from build123d import *

# Parameters (mm, degrees)
ESQUISSE1_R      = 4
EXTRUSION1_DEPTH = 6
CONG_1_R         = 0.5


with BuildPart() as part:
    # Esquisse1 → Extrusion1 (new body)
    with BuildSketch(Plane.XY):
        Polygon((7.505553499, 0), (3.75277675, 6.5), (-3.75277675, 6.5), (-7.505553499, 0), (-3.75277675, -6.5), (3.75277675, -6.5), align=None)
        Circle(ESQUISSE1_R, mode=Mode.SUBTRACT)
    extrude(amount=EXTRUSION1_DEPTH)

    # Congé1
    cong_1_edges = [part.edges().sort_by_distance(p)[0] for p in [
        (-4, 0, 0),
        (-4, 0, 6),
    ]]
    fillet(cong_1_edges, radius=CONG_1_R)


solid = part.part
Model file for the job. Use its own axes, mm. Give positions to 0.01 mm unless a question says otherwise; leave off trailing zeros. Loops run counter-clockwise (first coordinate to the right, second up) from the corner with the lowest first, then second, coordinate; pieces in that order, holes last. Notation, with made-up numbers: (32.25, 25) - (37.25, 25) arc R17 cw to (37.25, 36) - close; hole circle Ø7 at (2, 9). An arc over 180 degrees is marked (long way). Use one line per item in the form item = value.
(1) Cut at B-B (z = 2.9). Give the cut face in (x, y).
Determined:
outline = (-7.51, 0) - (-3.75, -6.5) - (3.75, -6.5) - (7.51, 0) - (3.75, 6.5) - (-3.75, 6.5) - close; hole circle Ø8 at (0, 0)
(2) Cut at C-C (x = -6). Give the cut face in (y, z), then the cut area to 3 significant figures.
Determined:
outline = (-2.61, 0) - (2.61, 0) - (2.61, 6) - (-2.61, 6) - close
area = 31.3 mm^2
(3) Pull direction X, two halves, no side cores. Call faces 1 (the face through (1.6, 4.4, 6)), 2 (the face through (-0.867, -3.905, 2.965)), 3 (the face through (-5.66, -3.2, 2.96)): pulls with the +X half, pulls with the -X half, needs draft (parallel to the pull), parting line crosses it, or undercut.
Determined:
face_1 = needs draft
face_2 = undercut
face_3 = pulls with the -X half
(4) Drill centre lines: L1, parallel to Y at x = 0, z = 3.85; L2, parallel to X at y = -2, z = 5.2; L3, parallel to X at y = -3, z = 3.75. Where is each one in solid material? Low to high.
Determined:
L1 = -6.5 to -4, 4 to 6.5
L2 = -6.35 to -3.46, 3.46 to 6.35
L3 = -5.77 to -2.65, 2.65 to 5.77
(5) Cut at A-A (x = 0). Give the cut face in (y, z).
Determined:
outline = (-6.5, 0) - (-4.5, 0) arc R0.5 ccw to (-4, 0.5) - (-4, 5.5) arc R0.5 ccw to (-4.5, 6) - (-6.5, 6) - close; (4, 0.5) arc R0.5 ccw to (4.5, 0) - (6.5, 0) - (6.5, 6) - (4.5, 6) arc R0.5 ccw to (4, 5.5) - close
(6) Drop flat-ended pins along their axis: P1, Ø1, axis at x = -1, y = 2, coming from the +Z side; P2, Ø1, axis at x = -6, y = 3.5, coming from the -Z side. Give the stop position or say it passes through.
Determined:
P1 = through
P2 = 0
